Build history of the part. All positions in model axes, mm. Face numbers are marked on the shaded views. A direction names the side the tool comes from. Round coordinates to 2 decimals unless told otherwise and drop trailing zeros. Write each loop counter-clockwise with the first axis right and the second up, starting at its lowest first coordinate (ties: lowest second). Pieces come first, ordered by that corner, then holes. Notation, with made-up numbers: M 68,-17 L 76,-17 A15 ccw 76,0 Z; hole C 88,77.5 d2. An arc over 180 degrees is marked long. Write item = value, one per line. Start each with the question number.
Q1. Band-saw the part on B-B on y = 0. Write the cut outline in (x, z).
Q2. Band-saw the part on A-A on z = 0.5. Write the cut outline in (x, y).
Q3. Band-saw the part on C-C on x = 1.8. Write the cut outline in (y, z).
Q4. Drop a flat-ended pin along its axis: P1, Ø0.6, axis at x = 0, y = 0, coming from the -Z side. Give the stop position or say it passes through.
Q5. Probe L1, parallel to X at y = 0.1, z = 0.5; L2, parallel to Z at x = -1.75, y = -1.1; L3, parallel to X at y = -0.9, z = 0.5. List the from-to ranges inside material, lowest first.
Q6. Band-saw the part on D-D on z = 2.25. Write the cut outline in (x, y), plus the area to 3 significant figures.
Q7. Tool access for the marked faces 4, 5 and 6: list every direction of +Z, -Z, +X, -X, +Y, -Y with a clear straight run to the whole face (end or side of a thin tool).
Q8. Pull direction Y, two halves, no side cores. Call the marked faces 1, 2 and 3: released by +Y, released by -Y, zero draft, split by the parting line, or undercut.
```python
from build123d import *

# Parameters (mm, degrees)
SKETCH_1_R          = 2.25
EXTRUDE_1_DEPTH     = 2.5
SKETCH_2_R          = 1.25
EXTRUDE_2_DEPTH     = 4
CHAMFER_1_SIZE      = 0.2
CUT_EXTRUDE_1_DEPTH = 1.1


with BuildPart() as part:
    # 草图1 → 凸台-拉伸1 (new body)
    with BuildSketch(Plane.XY):
        Circle(SKETCH_1_R)
    extrude(amount=EXTRUDE_1_DEPTH)

    # 草图2 → 凸台-拉伸2 (add)
    with BuildSketch(Plane.XY.offset(2.5)):
        Circle(SKETCH_2_R)
    extrude(amount=EXTRUDE_2_DEPTH)

    # 倒角1
    chamfer_1_edges = [part.edges().sort_by_distance(p)[0] for p in [
        (-1.25, 0, 6.5),
    ]]
    chamfer(chamfer_1_edges, length=CHAMFER_1_SIZE)

    # 草图3 → 切除-拉伸1 (cut)
    with BuildSketch(Plane(origin=(0, 0, 0), x_dir=(-1, 0, 0), z_dir=(0, 0, -1))):
        Polygon((0, 1.177794549), (-1.02, 0.588897275), (-1.02, -0.588897275), (0, -1.177794549), (1.02, -0.588897275), (1.02, 0.588897275), align=None)
    extrude(amount=-CUT_EXTRUDE_1_DEPTH, mode=Mode.SUBTRACT)


solid = part.part
```
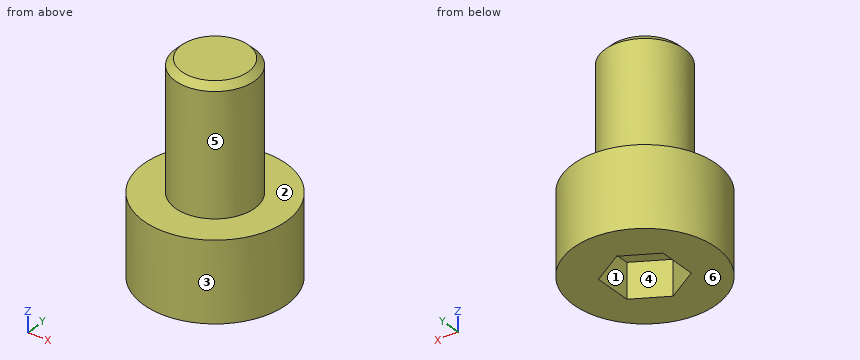
Conclusion:
q1.outline = M -2.25,0 L -1.02,0 L -1.02,1.1 L 1.02,1.1 L 1.02,0 L 2.25,0 L 2.25,2.5 L 1.25,2.5 L 1.25,6.3 L 1.05,6.5 L -1.05,6.5 L -1.25,6.3 L -1.25,2.5 L -2.25,2.5 Z
q2.outline = C 0,0 d4.5; hole M -1.02,-0.59 L 0,-1.18 L 1.02,-0.59 L 1.02,0.59 L 0,1.18 L -1.02,0.59 Z
q3.outline = M -1.35,0 L 1.35,0 L 1.35,2.5 L -1.35,2.5 Z
q4.P1 = 1.1
q5.L1 = -2.25 to -1.02, 1.02 to 2.25
q5.L2 = 0 to 2.5
q5.L3 = -2.06 to -0.48, 0.48 to 2.06
q6.outline = C 0,0 d4.5
q6.area = 15.9 mm^2
q7.face_4 = -Z
q7.face_5 = +Z
q7.face_6 = -Z, +X, -X, +Y, -Y
q8.face_1 = undercut
q8.face_2 = zero draft
q8.face_3 = split by the parting line
